Geometry: final body of the model. Coordinates: model frame, mm. Face numbers are marked on the shaded views. Give positions to 0.01 mm unless a question says otherwise; leave off trailing zeros. Write each loop counter-clockwise with the first axis right and the second up, starting at its lowest first coordinate (ties: lowest second). Pieces come first, ordered by that corner, then holes.
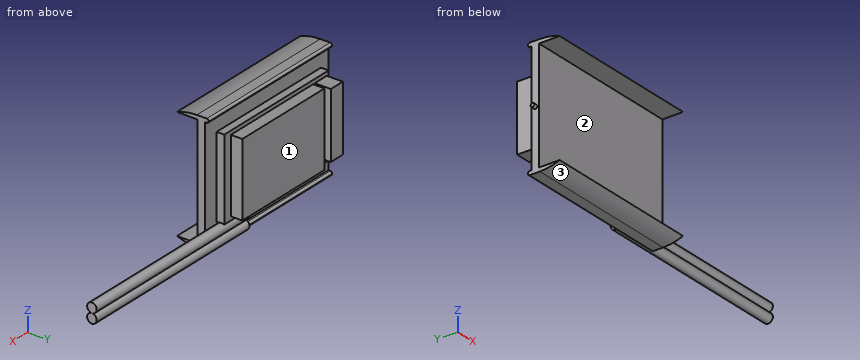
from build123d import *

# Parameters (mm, degrees)
SKETCH1_W               = 21
SKETCH1_H               = 15.6
BOSS_EXTRUDE1_DEPTH     = 0.95
SKETCH2_W               = 21
SKETCH2_H               = 0.5
BOSS_EXTRUDE2_DEPTH     = 2.7
FILLET1_R               = 7
SKETCH3_W               = 17.75
SKETCH3_H               = 10.6
BOSS_EXTRUDE3_DEPTH     = 1
SKETCH4_W               = 13.98
SKETCH4_H               = 9.6
BOSS_EXTRUDE4_DEPTH     = 2.5
SKETCH5_W               = 2.05
SKETCH5_H               = 8.6
BOSS_EXTRUDE5_DEPTH     = 3.1
SKETCH6_W               = 21
SKETCH6_H               = 0.5
BOSS_EXTRUDE6_DEPTH     = 0.5
FILLET2_R               = 0.25
BOSS_EXTRUDE9_START     = -7.66445529
BOSS_EXTRUDE9_OUTLINE_W = 26
BOSS_EXTRUDE9_OUTLINE_H = 0.1
BOSS_EXTRUDE9_DEPTH     = 2.36445529
BOSS_EXTRUDE9_START_2   = 4.5
BOSS_EXTRUDE9_2_DEPTH   = 26
SKETCH8_R               = 0.25
BOSS_EXTRUDE10_DEPTH    = 0.5


with BuildPart() as part:
    # Sketch1 → Boss-Extrude1 (new body)
    with BuildSketch(Plane(origin=(0, 0, 0), x_dir=(1, 0, 0), z_dir=(0, 1, 0))):
        Rectangle(SKETCH1_W, SKETCH1_H)
    extrude(amount=-BOSS_EXTRUDE1_DEPTH)

    # Sketch2 → Boss-Extrude2 (add)
    with BuildSketch(Plane.XZ.offset(0.95)):
        with Locations((0, 7.55)):
            Rectangle(SKETCH2_W, SKETCH2_H)
        with Locations((0, -7.55)):
            Rectangle(SKETCH2_W, SKETCH2_H)
    extrude(amount=BOSS_EXTRUDE2_DEPTH)

    # Fillet1
    # the kernel refuses this fillet: 7 mm, written as the material it takes off along each edge
    with BuildSketch(Plane(origin=(-16.995190528, -3.65, -7.8), x_dir=(0, 1, 0), z_dir=(1, 0, 0))) as fillet1_piece_1:
        with BuildLine():
            CenterArc((2.598076211, 7), FILLET1_R, 248.213210702, 21.786789298)
            Line((0, 0.5), (0, 0))
            Line((0, 0), (2.598076211, 0))
        make_face()
    extrude(amount=33.990381057, mode=Mode.SUBTRACT)
    with BuildSketch(Plane(origin=(-16.995190528, -3.65, 7.8), x_dir=(0, 1, 0), z_dir=(1, 0, 0))) as fillet1_piece_2:
        with BuildLine():
            CenterArc((2.598076211, -7), FILLET1_R, 90, 21.786789298)
            Line((0, -0.5), (0, 0))
            Line((0, 0), (2.598076211, 0))
        make_face()
    extrude(amount=33.990381057, mode=Mode.SUBTRACT)

    # Sketch3 → Boss-Extrude3 (add)
    with BuildSketch(Plane(origin=(0, 0, 0), x_dir=(1, 0, 0), z_dir=(0, 1, 0))):
        with Locations((-0.375, 0)):
            Rectangle(SKETCH3_W, SKETCH3_H)
    extrude(amount=BOSS_EXTRUDE3_DEPTH)

    # Sketch4 → Boss-Extrude4 (add)
    with BuildSketch(Plane(origin=(0, 0, 0), x_dir=(1, 0, 0), z_dir=(0, 1, 0))):
        with Locations((0.39, 0)):
            Rectangle(SKETCH4_W, SKETCH4_H)
    extrude(amount=BOSS_EXTRUDE4_DEPTH)

    # Sketch5 → Boss-Extrude5 (add)
    with BuildSketch(Plane(origin=(0, 0, 0), x_dir=(1, 0, 0), z_dir=(0, 1, 0))):
        with Locations((-7.925, -0.5)):
            Rectangle(SKETCH5_W, SKETCH5_H)
    extrude(amount=BOSS_EXTRUDE5_DEPTH)

    # Sketch6 → Boss-Extrude6 (add)
    with BuildSketch(Plane(origin=(0, 0, 0), x_dir=(1, 0, 0), z_dir=(0, 1, 0))):
        with Locations((0, 7.55)):
            Rectangle(SKETCH6_W, SKETCH6_H)
        with Locations((0, -7.55)):
            Rectangle(SKETCH6_W, SKETCH6_H)
    extrude(amount=BOSS_EXTRUDE6_DEPTH)

    # Fillet2
    fillet2_edges = [part.edges().sort_by_distance(p)[0] for p in [
        (0, 0.5, 7.8),
        (0, 0.5, 7.3),
        (0, 0.5, -7.3),
        (0, 0.5, -7.8),
    ]]
    fillet(fillet2_edges, radius=FILLET2_R - 0.0001)  # a hair under: the kernel refuses the full size

    # Boss-Extrude9: read off the stored shape, not the designer's step
    # Boss-Extrude9 outline → Boss-Extrude9 (add)
    with BuildSketch(Plane.XY.offset(BOSS_EXTRUDE9_START)):
        with Locations((17.5, 0.64)):
            Rectangle(BOSS_EXTRUDE9_OUTLINE_W, BOSS_EXTRUDE9_OUTLINE_H)
    extrude(amount=BOSS_EXTRUDE9_DEPTH)

    # Boss-Extrude9 2 outline → Boss-Extrude9 2 (add)
    with BuildSketch(Plane.YZ.offset(BOSS_EXTRUDE9_START_2)):
        with BuildLine():
            Line((0.69, -5.3), (0.69, -6.468486055))
            ThreePointArc((0.69, -6.468486055), (0.559870848, -5.22628961), (0.59, -6.474919995))
            Line((0.59, -6.474919995), (0.59, -5.3))
            Line((0.59, -5.3), (0.69, -5.3))
        make_face()
        with BuildLine():
            Line((0.69, -6.481513945), (0.69, -7.66445529))
            Line((0.69, -7.66445529), (0.59, -7.66445529))
            Line((0.59, -7.66445529), (0.59, -6.475080005))
            ThreePointArc((0.59, -6.475080005), (0.559870848, -7.72371039), (0.69, -6.481513945))
        make_face()
    extrude(amount=BOSS_EXTRUDE9_2_DEPTH)

    # Sketch8 → Boss-Extrude10 (add)
    with BuildSketch(Plane.ZY.offset(10.5)):
        with Locations((0, -0.485546963)):
            Circle(SKETCH8_R)
    extrude(amount=BOSS_EXTRUDE10_DEPTH)


solid = part.part
Q1. Section C-C on y = -2.5. Output: boundary loops of the cut face in (x, z), plus the area to 3 significant figures.
Filled sheet:
outline: (-10.5, -7.65) - (10.5, -7.65) - (10.5, -7.3) - (-10.5, -7.3) - close; (-10.5, 7.3) - (10.5, 7.3) - (10.5, 7.65) - (-10.5, 7.65) - close
area: 14.6 mm2
Q2. Pin query (flat end, axial travel): P1, Ø5, axis at x = 14.5, z = 0.5, coming from the -Y side; P2, Ø1, axis at y = 2, z = -1, coming from the -X side; P3, Ø7.5, axis at x = 4, z = 2, coming from the -Y side; P4, Ø0.6, axis at x = -8, y = 2, coming from the -Z side. Return the tip coordinate at first contact, or that it passes through.
Filled sheet:
P1: passes through
P2: stops at x = -8.95
P3: stops at y = -0.95
P4: stops at z = -3.8
Q3. Ray query, line 1 along Z through (x, y) = (9, 0.25); line 2 along Y through (x, z) = (5.5, -1.5); line 3 along Z through (x, y) = (3, 0.75). Return the intervals inside material, ascending.
Filled sheet:
line 1: z = -7.8 to -6.58, -6.37 to -5.33, 7.3 to 7.8
line 2: y = -0.95 to 2.5
line 3: z = -5.3 to 5.3
Q4. Pull-direction query (Z, two-part tool) for the marked faces 1, 2 and 3; classes: released by +Z, released by -Z, zero draft, split by the parting line, or undercut.
Filled sheet:
face 1: zero draft
face 2: undercut
face 3: released by -Z
Q5. Section A-A on y = 2. Output: boundary loops of the cut face in (x, z).
Filled sheet:
outline: (-8.95, -3.8) - (-6.9, -3.8) - (-6.9, 4.8) - (-8.95, 4.8) - close; (-6.6, -4.8) - (7.38, -4.8) - (7.38, 4.8) - (-6.6, 4.8) - close
